Drawing for the job (mm, zero at the part's lowest x, y, z). A direction names the side the tool comes from. Round coordinates to 2 decimals unless told otherwise and drop trailing zeros. Loops run counter-clockwise (first coordinate to the right, second up) from the corner with the lowest first, then second, coordinate; pieces in that order, holes last. Notation, with made-up numbers: M 20,81 L 76,81 A17 cw 76,94 Z; hole C 73.25,36.5 d5. An arc over 180 degrees is marked long. Put each result on its own line as item: value. Start each with the question number.
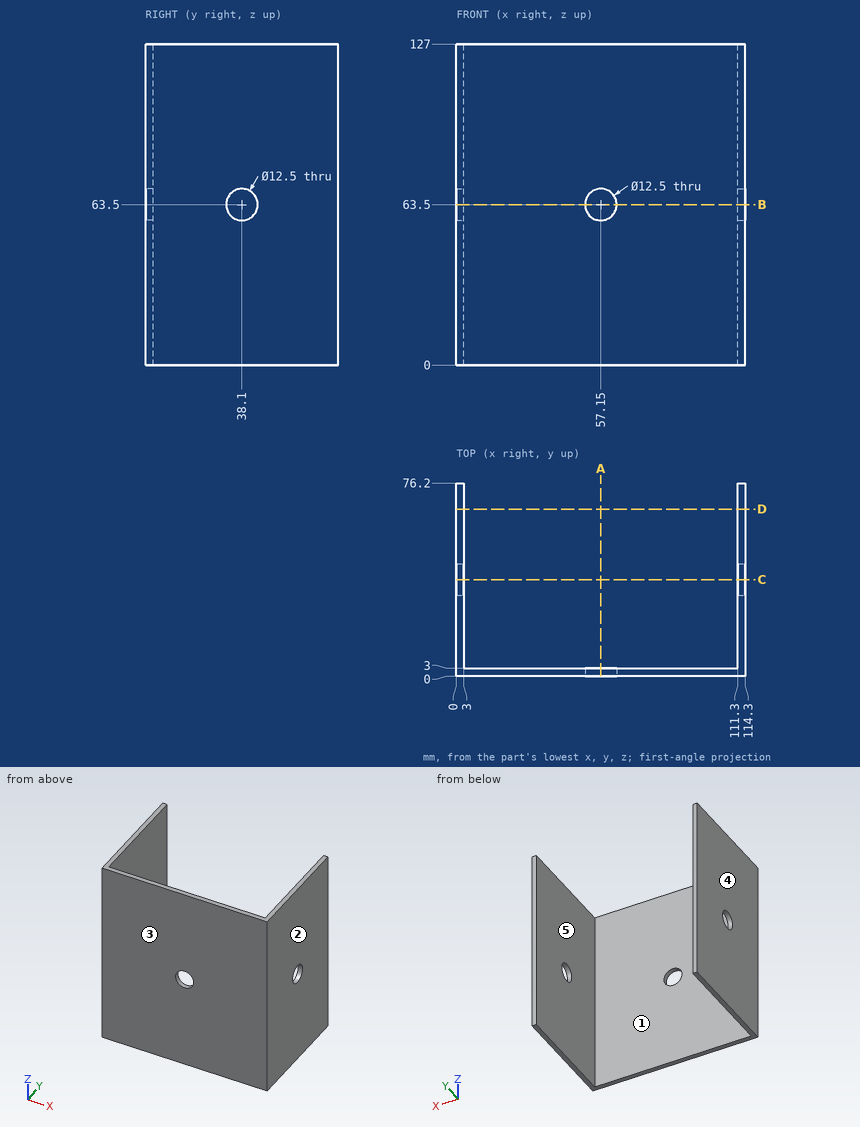
1. Cut at B-B, the plane z = 63.5. Give the cut face in (x, y).
2. Cut at A-A, the plane x = 57.15. Give the cut face in (y, z).
3. Drop flat-ended pins along their axis: pin 1 (14.5 mm diameter, centred on x = 57.15, z = 63.5, fed in from +Y); pin 2 (20 mm diameter, centred on y = 38.1, z = 63.5, fed in from -X). Give the stop position or say it passes through.
4. Mould opens along X. For the marked faces 3, 4 and 5 say: released by +X, released by -X, zero draft, split by the parting line, or undercut.
5. Wall check: L1, parallel to X at y = 1, z = 63; L2, parallel to X at y = 61.5, z = 61.5; L3, parallel to Y at x = 97.5, z = 92. Give the ranges that are in metal, low to high.
6. Cut at D-D, the plane y = 66. Give the cut face in (x, z), and give its area (3 significant figures).
7. Cut at C-C, the plane y = 38.1. Give the cut face in (x, z), and give its area (3 significant figures).
8. Which spindle directions (+Z, -Z, +X, -X, +Y, -Y) get a long thin tool onto all of the face, cutting with end or side? Do the marked faces 1 and 2. Say none if no direction does.
Results list:
1. outline: M 0,0 L 50.9,0 L 50.9,3 L 3,3 L 3,31.85 L 0,31.85 Z; M 0,44.35 L 3,44.35 L 3,76.2 L 0,76.2 Z; M 63.4,0 L 114.3,0 L 114.3,31.85 L 111.3,31.85 L 111.3,3 L 63.4,3 Z; M 111.3,44.35 L 114.3,44.35 L 114.3,76.2 L 111.3,76.2 Z
2. outline: M 0,0 L 3,0 L 3,57.25 L 0,57.25 Z; M 0,69.75 L 3,69.75 L 3,127 L 0,127 Z
3. pin 1: stops at y = 3
3. pin 2: stops at x = 0
4. face 3: zero draft
4. face 4: released by -X
4. face 5: undercut
5. L1: x = 0 to 50.92, 63.38 to 114.3
5. L2: x = 0 to 3, 111.3 to 114.3
5. L3: y = 0 to 3
6. outline: M 0,0 L 3,0 L 3,127 L 0,127 Z; M 111.3,0 L 114.3,0 L 114.3,127 L 111.3,127 Z
6. area: 762 mm^2
7. outline: M 0,0 L 3,0 L 3,57.25 L 0,57.25 Z; M 0,69.75 L 3,69.75 L 3,127 L 0,127 Z; M 111.3,0 L 114.3,0 L 114.3,57.25 L 111.3,57.25 Z; M 111.3,69.75 L 114.3,69.75 L 114.3,127 L 111.3,127 Z
7. area: 687 mm^2
8. face 1: +Z, -Z, +Y
8. face 2: +Z, -Z, +X, +Y, -Y
